Can you work these out from the model? Positions are in its coordinate system, mm. A direction names the side the tool comes from. Round coordinates to 2 decimals unless told otherwise and drop trailing zeros. Loops run counter-clockwise (first coordinate to the right, second up) from the corner with the lowest first, then second, coordinate; pieces in that order, holes last. Notation, with made-up numbers: (89, -30.75) -> (100, -30.75) arc R25 cw to (100, -17.75) -> close; hole circle Ø1 at (29.25, 56.25). An arc over 180 degrees is marked (long way). Answer as a JSON object with one key per item and string values.
```python
from build123d import *

# Parameters (mm, degrees)
SKETCH2_W           = 4
SKETCH2_H           = 4
BOSS_EXTRUDE1_DEPTH = 4
FILLET1_R           = 1
SKETCH3_R           = 1.5
BOSS_EXTRUDE2_DEPTH = 9.8


with BuildPart() as part:
    # Sketch2 → Boss-Extrude1 (new body)
    with BuildSketch(Plane(origin=(0, 0, 0), x_dir=(0, 0, -1), z_dir=(1, 0, 0))):
        with Locations((2, 2)):
            Rectangle(SKETCH2_W, SKETCH2_H)
    extrude(amount=BOSS_EXTRUDE1_DEPTH)

    # Fillet1
    fillet1_edges = [part.edges().sort_by_distance(p)[0] for p in [
        (4, 2, -4),
        (0, 2, -4),
    ]]
    fillet(fillet1_edges, radius=FILLET1_R)

    # Sketch3 → Boss-Extrude2 (add)
    with BuildSketch(Plane.XY):
        with Locations((2, 2)):
            Circle(SKETCH3_R)
    extrude(amount=BOSS_EXTRUDE2_DEPTH)


solid = part.part
```
Q1. I want a section at B-B, the plane y = 2. Write out the boundary of the cut face in (x, z), then the cut area to 3 significant figures.
Determined:
{"outline": "(0, -3) arc R1 ccw to (1, -4) -> (3, -4) arc R1 ccw to (4, -3) -> (4, 0) -> (3.5, 0) -> (3.5, 9.8) -> (0.5, 9.8) -> (0.5, 0) -> (0, 0) -> close", "area": "45.0 mm²"}
Q2. I want a section at A-A, the plane x = 2. Write out the boundary of the cut face in (y, z).
Determined:
{"outline": "(0, -4) -> (4, -4) -> (4, 0) -> (3.5, 0) -> (3.5, 9.8) -> (0.5, 9.8) -> (0.5, 0) -> (0, 0) -> close"}
Q3. I'm going to push flat-ended pins straight in: pin 1 (1.5 mm diameter, centred on x = 1.5, z = 2.5, fed in from -Y); pin 2 (2 mm diameter, centred on y = 3.5, z = 4, fed in from -X); pin 3 (2 mm diameter, centred on y = 3, z = 7, fed in from -X). Where does each tip first touch, or does it pass through?
Determined:
{"pin 1": "y = 0.5", "pin 2": "x = 0.59", "pin 3": "x = 0.5"}
Q4. If I drill on L1, parallel to Z at x = 2.75, y = 0.3; L2, parallel to X at y = 2.85, z = 0.75; L3, parallel to Z at x = 0.45, y = 2.05, over which ranges is the centre line in solid material (lowest first)? Write a range as [from, to].
Determined:
{"L1": "[-4, 0]", "L2": "[0.76, 3.24]", "L3": "[-3.84, 0]"}
Q5. On a 3-axis mill with a long thin cutter (end or side, diameter ignored), from which of +Z, -Z, +X, -X, +Y, -Y can I reach the whole of each face in a straight line? I mean faces 1 (the flat face through (2, 4, -2)), 2 (the cylindrical face through (0.8, 1.1, 4.8)). Say none if no direction works.
Determined:
{"face 1": "+Z, -Z, +X, -X, +Y", "face 2": "+Z"}
Q6. I want a section at C-C, the plane z = 6. Write out the boundary of the cut face in (x, y), then the cut area to 3 significant figures.
Determined:
{"outline": "circle Ø3 at (2, 2)", "area": "7.07 mm²"}
Q7. I want a section at D-D, the plane y = 2.85. Write out the boundary of the cut face in (x, z).
Determined:
{"outline": "(0, -3) arc R1 ccw to (1, -4) -> (3, -4) arc R1 ccw to (4, -3) -> (4, 0) -> (3.24, 0) -> (3.24, 9.8) -> (0.76, 9.8) -> (0.76, 0) -> (0, 0) -> close"}
